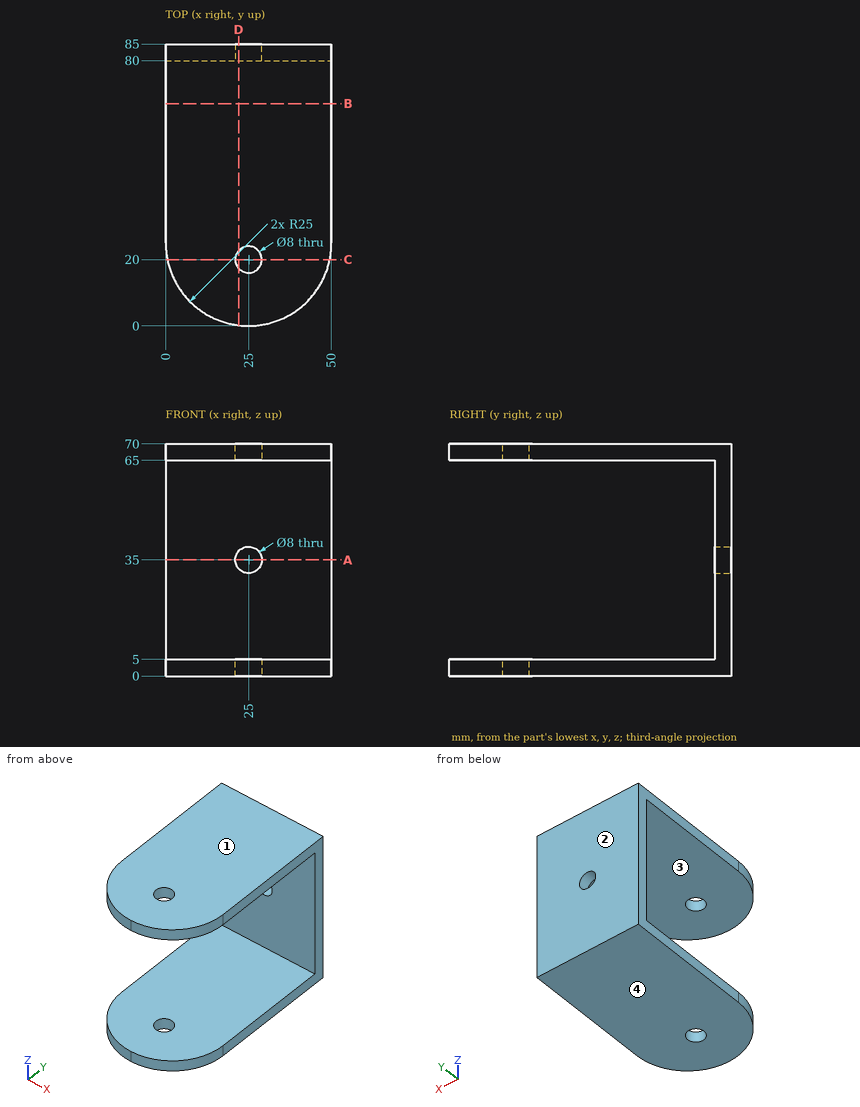
Verification items for this drawing (mm, ordinates from the low corner). Coordinates: 2 decimals unless noted, no trailing zeros. Order: outer loops, then holes, each group sorted by start corner. A loop starts at its lowest first (then second) coordinate and runs counter-clockwise, first axis right, second up. Notation, with made-up numbers: (13, 41.5) - (53, 41.5) arc R23 ccw to (53, 66.5) - close; hole circle Ø1 at (-18, 26.25). An arc over 180 degrees is marked (long way). Use one line per item in the form item = value.
1. Section check A-A (z = 35). Record the boundary of the cut face in (x, y).
Here are the results:
outline = (0, 80) - (21, 80) - (21, 85) - (0, 85) - close; (29, 80) - (50, 80) - (50, 85) - (29, 85) - close
2. Gauge pin test, flat end, axial feed: pin 1 (10 mm diameter, centred on x = 39, z = 46.5, fed in from -Y). Record the tip position at first contact, or that the pin passes through.
Here are the results:
pin_1 = 80
3. Section check C-C (y = 20). Record the boundary of the cut face in (x, z) (3 decimals), then the cut area to 3 significant figures.
Here are the results:
outline = (0.505, 0) - (21, 0) - (21, 5) - (0.505, 5) - close; (0.505, 65) - (21, 65) - (21, 70) - (0.505, 70) - close; (29, 0) - (49.495, 0) - (49.495, 5) - (29, 5) - close; (29, 65) - (49.495, 65) - (49.495, 70) - (29, 70) - close
area = 410 mm²
4. Section check B-B (y = 67). Record the boundary of the cut face in (x, z).
Here are the results:
outline = (0, 0) - (50, 0) - (50, 5) - (0, 5) - close; (0, 65) - (50, 65) - (50, 70) - (0, 70) - close
5. Scan lines: line 1 (Z direction, x = 6, y = 21.5); line 2 (Z direction, x = 25, y = 82.8); line 3 (Y direction, x = 25, z = 68.05). Record each from-to range of solid material in increasing order.
Here are the results:
line_1 = 0 to 5, 65 to 70
line_2 = 0 to 31, 39 to 70
line_3 = 0 to 16, 24 to 85
6. Section check D-D (x = 22). Record the boundary of the cut face in (y, z), then the cut area to 3 significant figures.
Here are the results:
outline = (0.18, 0) - (17.35, 0) - (17.35, 5) - (0.18, 5) - close; (0.18, 65) - (17.35, 65) - (17.35, 70) - (0.18, 70) - close; (22.65, 0) - (85, 0) - (85, 32.35) - (80, 32.35) - (80, 5) - (22.65, 5) - close; (22.65, 65) - (80, 65) - (80, 37.65) - (85, 37.65) - (85, 70) - (22.65, 70) - close
area = 1,070 mm²
7. Draft check along Z on the marked faces 1, 2, 3 and 4. Enter one of: pulls with the +Z half, pulls with the -Z half, needs draft (parallel to the pull), parting line crosses it, or undercut.
Here are the results:
face_1 = pulls with the +Z half
face_2 = needs draft
face_3 = undercut
face_4 = pulls with the -Z half
